```python
from build123d import *

# Parameters (mm, degrees)
TOP_R              = 12.5
MIDDLE_R           = 16.25
INSIDE_TOP_R       = 11.25
INSIDE_BOTTOM_R    = 15
ZAOKR_GLENIE1_R    = 1
ZAOKR_GLENIE2_R    = 1.5
LATCH_START        = -9
LATCH_DEPTH        = 9.75
LATCH_CUTOUT_DEPTH = 6
SZYK_KO_OWY2_COUNT = 3


with BuildPart() as part:
    # top → outside section 0
    with BuildSketch(Plane.XY):
        Circle(TOP_R)
    # middle → outside section 1
    with BuildSketch(Plane.XY.offset(-8.5)):
        Circle(MIDDLE_R)
    loft()

    # inside-top → inside-cutout section 0
    with BuildSketch(Plane.XY.offset(-1.5)):
        Circle(INSIDE_TOP_R)
    # inside-bottom → inside-cutout section 1
    with BuildSketch(Plane.XY.offset(-8.5)):
        Circle(INSIDE_BOTTOM_R)
    loft(mode=Mode.SUBTRACT)

    # Zaokrąglenie1
    zaokr_glenie1_edges = [part.edges().sort_by_distance(p)[0] for p in [
        (-11.25, 0, -1.5),
    ]]
    fillet(zaokr_glenie1_edges, radius=ZAOKR_GLENIE1_R)

    # Zaokrąglenie2
    zaokr_glenie2_edges = [part.edges().sort_by_distance(p)[0] for p in [
        (-12.5, 0, 0),
    ]]
    fillet(zaokr_glenie2_edges, radius=ZAOKR_GLENIE2_R)

    # Szkic6 → latch (add)
    with BuildSketch(Plane.XY.offset(-5).offset(LATCH_START)):
        Polygon((12.5, 0), (12.5, -3), (14, -3), (14, 3), (12.5, 3), align=None)
    latch = extrude(amount=LATCH_DEPTH)

    # Szkic → latch-cutout (cut)
    with BuildSketch(Plane(origin=(0, -3, 0), x_dir=(-1, 0, 0), z_dir=(0, -1, 0))):
        Polygon((-14, 9.7), (-13, 9.7), (-13, 8.2), (-14, 8.2), (-14.5, 8.2), (-14.5, 14), (-14, 14), (-13, 14), align=None)
    latch_cutout = extrude(amount=-LATCH_CUTOUT_DEPTH, mode=Mode.SUBTRACT)

    # Szyk kołowy2: latch, latch-cutout ×3 about axis
    szyk_ko_owy2_axis = Axis((0, 0, 0), (0, 0, 1))
    add([latch.rotate(szyk_ko_owy2_axis, i * 360 / SZYK_KO_OWY2_COUNT) for i in range(1, SZYK_KO_OWY2_COUNT)])
    add([latch_cutout.rotate(szyk_ko_owy2_axis, i * 360 / SZYK_KO_OWY2_COUNT) for i in range(1, SZYK_KO_OWY2_COUNT)], mode=Mode.SUBTRACT)


solid = part.part
```
Source: CAD feature listing. Evaluate the final solid. Frame: model axes, mm. A direction names the side the tool comes from. Round coordinates to 2 decimals unless told otherwise and drop trailing zeros. Loops run counter-clockwise (first coordinate to the right, second up) from the corner with the lowest first, then second, coordinate; pieces in that order, holes last. Notation, with made-up numbers: M -8,25 L 39,25 A22 ccw 39,54 Z; hole C 4.25,36.25 d1. An arc over 180 degrees is marked long. Put each result on its own line as item: value.
(1) Section B-B, the plane x = 0. Return loops of the section in (y, z).
Solutions:
outline: M -16.25,-8.5 L -15,-8.5 L -11.53,-2.03 A1 cw -10.65,-1.5 L 10.65,-1.5 A1 cw 11.53,-2.03 L 15,-8.5 L 16.25,-8.5 L 12.89,-0.89 A1.5 ccw 11.52,0 L -11.52,0 A1.5 ccw -12.89,-0.89 Z
(2) Section D-D, the plane z = -5.75. Return loops of the section in (x, y), and give its area (3 significant figures).
Solutions:
outline: C 0,0 d30.07; hole M -9.19,-9.92 L -8.85,-9.33 L -3.65,-12.33 L -4,-12.92 A13.53 ccw 13.19,-3 L 12.5,-3 L 12.5,3 L 13.19,3 A13.53 ccw -4,12.92 L -3.65,12.33 L -8.85,9.33 L -9.19,9.92 A13.53 ccw Z
area: 152 mm²
(3) Access query for faces 4 (the face through (-8.968, -9.533, -9.314)), 5 (the face through (13.493, -0.042, -11.88)), 6 (the face through (-6.46, 11.28, -8.96)). Directions: +Z, -Z, +X, -X, +Y, -Y. A direction counts if a zero-diameter tool reaches every point of the face in a straight line with its end or side. Return the directions, or none.
Solutions:
face 4: -Z
face 5: -Z, +X, +Y, -Y
face 6: none
(4) Ray query, line 1 (Y direction, x = -4, z = -7); line 2 (Z direction, x = -3, y = 0); line 3 (X direction, y = -11, z = -6.75). Return the intervals inside material, ascending. Write a range as [from, to].
Solutions:
line 1: [-15.07, -13.62], [-12.93, -12.12], [12.12, 12.93], [13.62, 15.07]
line 2: [-1.5, 0]
line 3: [-10.89, -5.95], [8.76, 10.89]
(5) First-contact query: pin 1 (0.7 mm diameter, centred on x = -5, y = 11.5, fed in from +Z); pin 2 (2 mm diameter, centred on x = 11.5, y = -7, fed in from +Z); pin 3 (6 mm diameter, centred on y = -5.5, z = -3.5, fed in from +X). Flat tips, straight axial feed; report the tip coordinate or a pass-through.
Solutions:
pin 1: z = -0.16
pin 2: z = -0.33
pin 3: x = 14.65
(6) Pull-direction query (Z, two-part tool) for faces 1 (the face through (13.5, 0, -8.2)), 2 (the face through (-3.78, -12.55, -9.31)), 3 (the face through (-6.783, -11.664, -11.88)); classes: released by +Z, released by -Z, zero draft, split by the parting line, or undercut.
Solutions:
face 1: undercut
face 2: zero draft
face 3: released by -Z
(7) Section A-A, the plane z = -7.75. Return loops of the section in (x, y), and give its area (3 significant figures).
Solutions:
outline: C 0,0 d31.84; M -9.6,-10.62 L -4.4,-13.62 L -3.65,-12.33 L -8.85,-9.33 Z; M -9.6,10.62 L -8.85,9.33 L -3.65,12.33 L -4.4,13.62 Z; M 12.5,-3 L 14,-3 L 14,3 L 12.5,3 Z; hole C 0,0 d29.2
area: 154 mm²
(8) Section C-C, the plane z = -12. Return loops of the section in (x, y), and give its area (3 significant figures).
Solutions:
outline: M -9.33,-10.16 L -4.13,-13.16 L -3.65,-12.33 L -8.85,-9.33 Z; M -9.33,10.16 L -8.85,9.33 L -3.65,12.33 L -4.13,13.16 Z; M 12.5,-3 L 13.47,-3 L 13.47,3 L 12.5,3 Z
area: 17.4 mm²
